```python
from build123d import *

# Parameters (mm, degrees)
AUFSATZ_LINEAR_AUSTRAGEN1_DEPTH                      = 230
STIRNSENKUNG_F_R_M6_ZYLINDERSCHRAUBE_MIT_D           = 6.6
STIRNSENKUNG_F_R_M6_ZYLINDERSCHRAUBE_MIT_CBORE_D     = 11
STIRNSENKUNG_F_R_M6_ZYLINDERSCHRAUBE_MIT_CBORE_DEPTH = 106.4


with BuildPart() as part:
    # Skizze1 → Aufsatz-Linear austragen1 (new body)
    with BuildSketch(Plane.XY):
        with BuildLine():
            Line((0, 104.095532512), (0, 0))
            Line((0, 0), (143.799350711, 0))
            ThreePointArc((143.799350711, 0), (145.702786731, 1.386052676), (144.967960163, 3.623068683))
            Line((144.967960163, 3.623068683), (3.168609452, 105.718601195))
            ThreePointArc((3.168609452, 105.718601195), (1.088193799, 105.875591346), (0, 104.095532512))
        make_face()
    extrude(amount=-AUFSATZ_LINEAR_AUSTRAGEN1_DEPTH)

    # Stirnsenkung für M6 Zylinderschraube mit Innensechskant1 (through all)
    with Locations(Plane(origin=(150, 0, 0), x_dir=(0, 0, -1), z_dir=(1, 0, 0))):
        with Locations((15, 50), (115, 50), (215, 50)):
            CounterBoreHole(STIRNSENKUNG_F_R_M6_ZYLINDERSCHRAUBE_MIT_D / 2, STIRNSENKUNG_F_R_M6_ZYLINDERSCHRAUBE_MIT_CBORE_D / 2, STIRNSENKUNG_F_R_M6_ZYLINDERSCHRAUBE_MIT_CBORE_DEPTH)


solid = part.part
```
Model file for the job. Use its own axes, mm. A direction names the side the tool comes from. Round coordinates to 2 decimals unless told otherwise and drop trailing zeros. Loops run counter-clockwise (first coordinate to the right, second up) from the corner with the lowest first, then second, coordinate; pieces in that order, holes last. Notation, with made-up numbers: M 22,15 L 31,15 A6 ccw 31,25 Z; hole C -23,82.25 d9. An arc over 180 degrees is marked long. Put each result on its own line as item: value. Start each with the question number.
Item 1: Cut at B-B (z = -115). List the corners of the cut face in (x, y), then the cut area to 3 significant figures.
Item 2: Drop flat-ended pins along their axis: P1, Ø9, axis at y = 47.5, z = -12.5, coming from the +X side; P2, Ø12, axis at y = 51, z = -213, coming from the +X side; P3, Ø8, axis at x = 112.5, z = -185, coming from the +Y side. Give the stop position or say it passes through.
Item 3: Cut at D-D (x = 119). List the corners of the cut face in (y, z), then the cut area to 3 significant figures.
Item 4: Drill centre lines: line 1 along Z through (x, y) = (55, 50); line 2 along Y through (x, z) = (23.5, -115); line 3 along X through (y, z) = (21.5, -103). Where is each one in solid material? Low to high.
Item 5: Mould opens along Y. For faces 3 (the face through (56, 42, 0)), 4 (the face through (71, 0, -113)), 5 (the face through (61.3, 45.1, -17.5)), 6 (the face through (61.33, 44.63, -213.81)) say: released by +Y, released by -Y, zero draft, split by the parting line, or undercut.
Item 6: Cut at A-A (y = 50). List the corners of the cut face in (x, z), then the cut area to 3 significant figures.
Item 7: Cut at C-C (z = -206). List the corners of the cut face in (x, y).
Item 8: 3-axis set-ups, long thin cutter, end or side, ignore diameter. For faces 1 (the face through (21.49, 52.23, -117.43)), 2 (the face through (43.6, 50, -19)): which of +Z, -Z, +X, -X, +Y, -Y reach the whole face in a straight line?
Answer block:
1. outline: M 0,0 L 143.8,0 A2 ccw 144.97,3.62 L 88.19,44.5 L 43.6,44.5 L 43.6,46.7 L 0,46.7 Z; M 0,53.3 L 43.6,53.3 L 43.6,55.5 L 72.92,55.5 L 3.17,105.72 A2 ccw 0,104.1 Z
1. area: 7,390 mm2
2. P1: x = 90.28
2. P2: x = 87.49
2. P3: y = 29.88
3. outline: M 0,-230 L 22.32,-230 L 22.32,0 L 0,0 Z
3. area: 5,130 mm2
4. line 1: -230 to -220.5, -209.5 to -120.5, -109.5 to -20.5, -9.5 to 0
4. line 2: 0 to 46.7, 53.3 to 91.08
4. line 3: 0 to 120.14
5. face 3: zero draft
5. face 4: released by -Y
5. face 5: undercut
5. face 6: undercut
6. outline: M 0,-230 L 80.56,-230 L 80.56,-220.5 L 43.6,-220.5 L 43.6,-218.3 L 0,-218.3 Z; M 0,-211.7 L 43.6,-211.7 L 43.6,-209.5 L 80.56,-209.5 L 80.56,-120.5 L 43.6,-120.5 L 43.6,-118.3 L 0,-118.3 Z; M 0,-111.7 L 43.6,-111.7 L 43.6,-109.5 L 80.56,-109.5 L 80.56,-20.5 L 43.6,-20.5 L 43.6,-18.3 L 0,-18.3 Z; M 0,-11.7 L 43.6,-11.7 L 43.6,-9.5 L 80.56,-9.5 L 80.56,0 L 0,0 Z
6. area: 16,400 mm2
7. outline: M 0,0 L 143.8,0 A2 ccw 144.97,3.62 L 3.17,105.72 A2 ccw 0,104.1 Z
8. face 1: +X, -X
8. face 2: +X
